from build123d import *

# Parameters (mm, degrees)
SALIENTE_EXTRUIR1_DEPTH = 22
CROQUIS2_R              = 19
SALIENTE_EXTRUIR2_DEPTH = 79
CROQUIS3_R              = 9.5
SALIENTE_EXTRUIR3_DEPTH = 2
SALIENTE_EXTRUIR4_DEPTH = 321
CROQUIS5_R              = 10
CORTAR_EXTRUIR1_DEPTH   = 321
SALIENTE_EXTRUIR5_DEPTH = 19
CORTAR_EXTRUIR2_REACH   = 354.007
CROQUIS8_R              = 3
REDONDEO1_R             = 1.5


with BuildPart() as part:
    # Croquis1 → Saliente-Extruir1 (new body)
    with BuildSketch(Plane.XY):
        with BuildLine():
            Line((-9, 0), (-30, 0))
            Line((-30, 0), (-39, 9))
            Line((-39, 9), (-39, 54.9875))
            ThreePointArc((-39, 54.9875), (-19.5, 74), (0, 54.9875))
            Line((0, 54.9875), (0, 9))
            Line((0, 9), (-9, 0))
        make_face()
    extrude(amount=SALIENTE_EXTRUIR1_DEPTH)

    # Croquis2 → Saliente-Extruir2 (add)
    with BuildSketch(Plane.XY.offset(22)):
        with Locations((-19.5, 54.5)):
            Circle(CROQUIS2_R)
    extrude(amount=SALIENTE_EXTRUIR2_DEPTH)

    # Croquis3 → Saliente-Extruir3 (add)
    with BuildSketch(Plane.XY.offset(101)):
        with Locations((-19.5, 54.5)):
            Circle(CROQUIS3_R)
    extrude(amount=SALIENTE_EXTRUIR3_DEPTH)

    # Croquis4 → Saliente-Extruir4 (add)
    with BuildSketch(Plane.XY.offset(22)):
        with BuildLine():
            Line((-32.5, 14), (-30, 0))
            Line((-30, 0), (-9, 0))
            Line((-9, 0), (-6.5, 14))
            ThreePointArc((-6.5, 14), (-19.5, 35.001407257), (-32.5, 14))
        make_face()
    extrude(amount=SALIENTE_EXTRUIR4_DEPTH)

    # Croquis5 → Cortar-Extruir1 (cut)
    with BuildSketch(Plane.XY.offset(343)):
        with Locations((-19.5, 20.001407257)):
            Circle(CROQUIS5_R)
    extrude(amount=-CORTAR_EXTRUIR1_DEPTH, mode=Mode.SUBTRACT)

    # Croquis6 → Saliente-Extruir5 (add)
    with BuildSketch(Plane(origin=(0, 0, 0), x_dir=(-1, 0, 0), z_dir=(0, 0, -1))):
        with BuildLine():
            Line((24, 11), (19.5, 11))
            Line((19.5, 11), (15, 11))
            ThreePointArc((15, 11), (12.171572875, 12.171572875), (11, 15))
            Line((11, 15), (11, 24))
            ThreePointArc((11, 24), (12.171572875, 26.828427125), (15, 28))
            Line((15, 28), (24, 28))
            ThreePointArc((24, 28), (26.828427125, 26.828427125), (28, 24))
            Line((28, 24), (28, 15))
            ThreePointArc((28, 15), (26.828427125, 12.171572875), (24, 11))
        make_face()
    extrude(amount=SALIENTE_EXTRUIR5_DEPTH)

    # Croquis8 → Cortar-Extruir2 (cut, up to next)
    with BuildSketch(Plane(origin=(-11, 0, 0), x_dir=(0, 0, -1), z_dir=(1, 0, 0)), mode=Mode.PRIVATE) as cortar_extruir2_sk1:
        with Locations(Location((11, 19.5, 0), (0, 0, 90))):
            Circle(CROQUIS8_R)
    cortar_extruir2_tool1 = extrude(cortar_extruir2_sk1.sketch, amount=-CORTAR_EXTRUIR2_REACH, mode=Mode.PRIVATE) & part.part
    add(cortar_extruir2_tool1.solids().sort_by_distance((-11, 19.5, -11))[0], mode=Mode.SUBTRACT)

    # Redondeo1
    redondeo1_edges = [part.edges().sort_by_distance(p)[0] for p in [
        (-11, 16.5, -11),
        (-28, 16.5, -11),
    ]]
    fillet(redondeo1_edges, radius=REDONDEO1_R - 0.0001)  # a hair under: the kernel refuses the full size


solid = part.part
The listing builds one solid part. Answer for the finished solid, in the listing's coordinates (mm). A direction names the side the tool comes from. Coordinates: 2 decimals unless noted, no trailing zeros. Order: outer loops, then holes, each group sorted by start corner. A loop starts at its lowest first (then second) coordinate and runs counter-clockwise, first axis right, second up. Notation, with made-up numbers: M -20,26.5 L -15,26.5 A36 cw -15,61.5 Z; hole C -9,-35 d11. An arc over 180 degrees is marked long. Use CSV: the item, a comma, the result in double quotes.
Q1. A tool of negligible diameter and unlimited length cuts with its end or side. For faces 1 (the flat face through (-11, 22, -7)), 2 (the flat face through (-20, 20, 22)), 3 (the flat face through (-28, 17, -7)), from which of +Z, -Z, +X, -X, +Y, -Y can it reach the whole face along a straight path? Write none if from no direction.
Here are the results:
face 1,"-Z, +X, +Y, -Y"
face 2,"+Z"
face 3,"-Z, -X, +Y, -Y"
Q2. Section D-D (z = 214) is taken. Determine the outline of the cut face in (x, y), then the cut area to 3 significant figures.
Here are the results:
outline,"M -32.5,14 L -30,0 L -9,0 L -6.5,14 A14.52 ccw long Z; hole C -19.5,20 d20"
area,"528 mm2"
Q3. Section B-B (z = 72.5) is taken. Determine the outline of the cut face in (x, y), then the cut area to 3 significant figures.
Here are the results:
outline,"C -19.5,54.5 d38; M -32.5,14 L -30,0 L -9,0 L -6.5,14 A14.52 ccw long Z; hole C -19.5,20 d20"
area,"1,660 mm2"
Q4. Given pin 1 Ø5.5 at (x, y) = (-16.5, 51.5) entering from +Z; pin 2 Ø18 at (x, y) = (-19.5, 20) entering from +Z; pin 3 Ø2.5 at (x, z) = (-18.5, -13.5) entering from -Y, each flat-ended and moving along its own axis, determine where each tip first touches the part or whether it passes through.
Here are the results:
pin 1,"z = 103"
pin 2,"z = 22"
pin 3,"y = 11"
Q5. Determine the mould class of faces 4 (the cylindrical face through (-19.087, 34.996, 180.253)), 5 (the cylindrical face through (-19.4, 16.5, -10.9)), 6 (the flat face through (-24, 63.2, 101)) for opening direction Z: pulls with the +Z half, pulls with the -Z half, needs draft (parallel to the pull), parting line crosses it, or undercut.
Here are the results:
face 4,"needs draft"
face 5,"undercut"
face 6,"pulls with the +Z half"
Q6. Straight lines are drawn through the part: L1, parallel to Y at x = -19, z = 176; L2, parallel to Z at x = -19.5, y = 19.5; L3, parallel to Y at x = -22, z = 70. For each, find the intervals that lie inside material, in ascending order.
Here are the results:
L1,"0 to 10.01, 29.99 to 34.99"
L2,"-19 to -14, -8 to 22"
L3,"0 to 10.32, 29.68 to 34.78, 35.67 to 73.33"
Q7. Section C-C (y = 67) is taken. Determine the outline of the cut face in (x, z), then the cut area to 3 significant figures.
Here are the results:
outline,"M -34.47,0 L -4.53,0 L -4.53,22 L -5.19,22 L -5.19,101 L -33.81,101 L -33.81,22 L -34.47,22 Z"
area,"2,920 mm2"
